Verification items for the finished model (mm, model axes). Face numbers are marked on the shaded views. A direction names the side the tool comes from. Coordinates: 2 decimals unless noted, no trailing zeros. Loops run counter-clockwise (first coordinate to the right, second up) from the corner with the lowest first, then second, coordinate; pieces in that order, holes last.
Q1. Access from +Z, -Z, +X, -X, +Y, -Y to the whole of each face (thin tool, end or side, straight path). Record for the marked faces 1, 2 and 3.
Q2. Sectioned sample at B-B (z = -46). Enter the section's corners in (x, y).
Q3. Go/stop test with flat-tipped pins: P1, Ø2, axis at y = -2.5, z = -36.5, coming from the -X side; P2, Ø16, axis at x = -39.5, z = -17.5, coming from the +Y side; P3, Ø13, axis at x = -18, y = 24.5, coming from the -Z side; P4, Ø1, axis at x = -24, y = 4.5, coming from the -Z side. Record where each tip stops, or that it passes through.
Q4. Sectioned sample at D-D (y = 12). Enter the section's corners in (x, z).
Q5. Sectioned sample at A-A (x = -46). Enter the section's corners in (y, z).
Q6. Material ranges on probe 1 along X at (y, z) = (-3.65, -46); probe 2 along Y at (x, z) = (-13, -16.5); probe 3 along Z at (x, y) = (-42, -2), recorded low to high.
Q7. Sectioned sample at C-C (x = -16.5). Enter the section's corners in (y, z).
```python
from build123d import *

# Parameters (mm, degrees)
SKETCH1_W                    = 33.7
SKETCH1_H                    = 20.3
SKETCH1_W_2                  = 20.3
SKETCH1_H_2                  = 33.7
BOSS_EXTRUDE1_DEPTH          = 24
SHELL1_T                     = -4
SKETCH2_R                    = 1
CUT_EXTRUDE1_DEPTH           = 24
SKETCH3_R                    = 4.2
CUT_EXTRUDE2_DEPTH           = 3
CUT_EXTRUDE2_DRAFT           = -45
CUT_EXTRUDE2_PROFILE_2_DEPTH = 3
CUT_EXTRUDE2_PROFILE_2_DRAFT = -45
SKETCH4_W                    = 20.3
SKETCH4_H                    = 22
BOSS_EXTRUDE2_DEPTH          = 50
SHELL2_T                     = -4
CUT_EXTRUDE3_REACH           = 93.28
SKETCH5_R                    = 1
SKETCH6_R                    = 4.2
CUT_EXTRUDE4_DEPTH           = 3
CUT_EXTRUDE4_DRAFT           = -45
CUT_EXTRUDE5_REACH           = 93.28
SKETCH7_R                    = 1
SKETCH8_R                    = 4.2
CUT_EXTRUDE6_DEPTH           = 3
CUT_EXTRUDE6_DRAFT           = -45
FILLET1_R                    = 10


with BuildPart() as part:
    # Sketch1 → Boss-Extrude1 (new body)
    with BuildSketch(Plane(origin=(0, 0, 0), x_dir=(1, 0, 0), z_dir=(0, 1, 0))):
        with Locations((-37.15, 10.15)):
            Rectangle(SKETCH1_W, SKETCH1_H)
        with Locations((-10.15, 10.15)):
            Rectangle(SKETCH1_W_2, SKETCH1_H)
        with Locations((-10.15, 37.15)):
            Rectangle(SKETCH1_W_2, SKETCH1_H_2)
    extrude(amount=-BOSS_EXTRUDE1_DEPTH)

    # Shell1
    shell1_openings = [part.faces().sort_by_distance(p)[0] for p in [
        (-53.236324676, -24, -10.15),
        (-54, -12, -10.15),
        (-37.15, -12, -20.3),
        (-20.3, -12, -37.15),
        (-10.15, -12, -54),
    ]]
    offset(amount=SHELL1_T, openings=shell1_openings, kind=Kind.INTERSECTION)

    # Sketch2 → Cut-Extrude1 (cut)
    with BuildSketch(Plane(origin=(0, 0, 0), x_dir=(1, 0, 0), z_dir=(0, 1, 0))):
        with Locations(Location((-10.15, 46, 0), (0, 0, 270))):
            Circle(SKETCH2_R)
        with Locations(Location((-46, 10.15, 0), (0, 0, 270))):
            Circle(SKETCH2_R)
    extrude(amount=-CUT_EXTRUDE1_DEPTH, mode=Mode.SUBTRACT)


with BuildPart() as cut_extrude2_tool:
    # Sketch3 → Cut-Extrude2 (with draft: the straight prism first)
    with BuildSketch(Plane(origin=(0, 0, 0), x_dir=(1, 0, 0), z_dir=(0, 1, 0))):
        with Locations((-46, 10.15)):
            Circle(SKETCH3_R)
    extrude(amount=-CUT_EXTRUDE2_DEPTH)
    # Cut-Extrude2: the draft: its side faces are tilted about the plane it starts from
    cut_extrude2_sides = [cut_extrude2_tool.faces().sort_by_distance(p)[0] for p in [
        (-50.2, -1.5, -10.15),
    ]]
    draft(cut_extrude2_sides, Plane(origin=(0, 0, 0), x_dir=(1, 0, 0), z_dir=(0, 1, 0)), CUT_EXTRUDE2_DRAFT)


with BuildPart() as part_1:
    add(part.part)

    # Cut-Extrude2: cut by cut_extrude2_tool
    add(cut_extrude2_tool.part, mode=Mode.SUBTRACT)


with BuildPart() as cut_extrude2_profile_2_tool:
    # Sketch3 → Cut-Extrude2 profile 2 (with draft: the straight prism first)
    with BuildSketch(Plane(origin=(0, 0, 0), x_dir=(1, 0, 0), z_dir=(0, 1, 0))):
        with Locations((-10.15, 46)):
            Circle(SKETCH3_R)
    extrude(amount=-CUT_EXTRUDE2_PROFILE_2_DEPTH)
    # Cut-Extrude2 profile 2: the draft: its side faces are tilted about the plane it starts from
    cut_extrude2_profile_2_sides = [cut_extrude2_profile_2_tool.faces().sort_by_distance(p)[0] for p in [
        (-14.35, -1.5, -46),
    ]]
    draft(cut_extrude2_profile_2_sides, Plane(origin=(0, 0, 0), x_dir=(1, 0, 0), z_dir=(0, 1, 0)), CUT_EXTRUDE2_PROFILE_2_DRAFT)


with BuildPart() as part_2:
    add(part_1.part)

    # Cut-Extrude2 profile 2: cut by cut_extrude2_profile_2_tool
    add(cut_extrude2_profile_2_tool.part, mode=Mode.SUBTRACT)


with BuildPart() as body_2:
    # Sketch4 → Boss-Extrude2 (new body)
    with BuildSketch(Plane(origin=(0, 0, 0), x_dir=(1, 0, 0), z_dir=(0, 1, 0))):
        with Locations((-10.15, 11)):
            Rectangle(SKETCH4_W, SKETCH4_H)
    extrude(amount=BOSS_EXTRUDE2_DEPTH)

    # Shell2
    shell2_openings = [body_2.faces().sort_by_distance(p)[0] for p in [
        (-10.15, 50, -11),
        (-10.15, 0, -11),
        (-20.3, 25, -11),
        (-10.15, 25, -22),
    ]]
    offset(amount=SHELL2_T, openings=shell2_openings, kind=Kind.INTERSECTION)


with BuildPart() as part_3:
    add(part_2.part)

    # Combine1: union body 2
    add(body_2.part)

    # Sketch5 → Cut-Extrude3 (cut, up to next)
    with BuildSketch(Plane.XY, mode=Mode.PRIVATE) as cut_extrude3_sk1:
        with Locations((-10.15, 42)):
            Circle(SKETCH5_R)
    cut_extrude3_tool1 = extrude(cut_extrude3_sk1.sketch, amount=-CUT_EXTRUDE3_REACH, mode=Mode.PRIVATE) & part_3.part
    add(cut_extrude3_tool1.solids().sort_by_distance((-10.15, 42, 0))[0], mode=Mode.SUBTRACT)


with BuildPart() as cut_extrude4_tool:
    # Sketch6 → Cut-Extrude4 (with draft: the straight prism first)
    with BuildSketch(Plane.XY):
        with Locations((-10.15, 42)):
            Circle(SKETCH6_R)
    extrude(amount=-CUT_EXTRUDE4_DEPTH)
    # Cut-Extrude4: the draft: its side faces are tilted about the plane it starts from
    cut_extrude4_sides = [cut_extrude4_tool.faces().sort_by_distance(p)[0] for p in [
        (-14.35, 42, -1.5),
    ]]
    draft(cut_extrude4_sides, Plane.XY, CUT_EXTRUDE4_DRAFT)


with BuildPart() as part_4:
    add(part_3.part)

    # Cut-Extrude4: cut by cut_extrude4_tool
    add(cut_extrude4_tool.part, mode=Mode.SUBTRACT)

    # Sketch7 → Cut-Extrude5 (cut, up to next)
    with BuildSketch(Plane(origin=(0, 0, 0), x_dir=(0, 0, -1), z_dir=(1, 0, 0)), mode=Mode.PRIVATE) as cut_extrude5_sk1:
        with Locations((11, 20)):
            Circle(SKETCH7_R)
    cut_extrude5_tool1 = extrude(cut_extrude5_sk1.sketch, amount=-CUT_EXTRUDE5_REACH, mode=Mode.PRIVATE) & part_4.part
    add(cut_extrude5_tool1.solids().sort_by_distance((0, 20, -11))[0], mode=Mode.SUBTRACT)


with BuildPart() as cut_extrude6_tool:
    # Sketch8 → Cut-Extrude6 (with draft: the straight prism first)
    with BuildSketch(Plane(origin=(0, 0, 0), x_dir=(0, 0, -1), z_dir=(1, 0, 0))):
        with Locations((11, 20)):
            Circle(SKETCH8_R)
    extrude(amount=-CUT_EXTRUDE6_DEPTH)
    # Cut-Extrude6: the draft: its side faces are tilted about the plane it starts from
    cut_extrude6_sides = [cut_extrude6_tool.faces().sort_by_distance(p)[0] for p in [
        (-1.5, 20, -6.8),
    ]]
    draft(cut_extrude6_sides, Plane(origin=(0, 0, 0), x_dir=(0, 0, -1), z_dir=(1, 0, 0)), CUT_EXTRUDE6_DRAFT)


with BuildPart() as part_5:
    add(part_4.part)

    # Cut-Extrude6: cut by cut_extrude6_tool
    add(cut_extrude6_tool.part, mode=Mode.SUBTRACT)

    # Fillet1
    fillet1_edges = [part_5.edges().sort_by_distance(p)[0] for p in [
        (-2, 0, -22),
        (-20.3, 0, -2),
    ]]
    fillet(fillet1_edges, radius=FILLET1_R)


solid = part_5.part
```
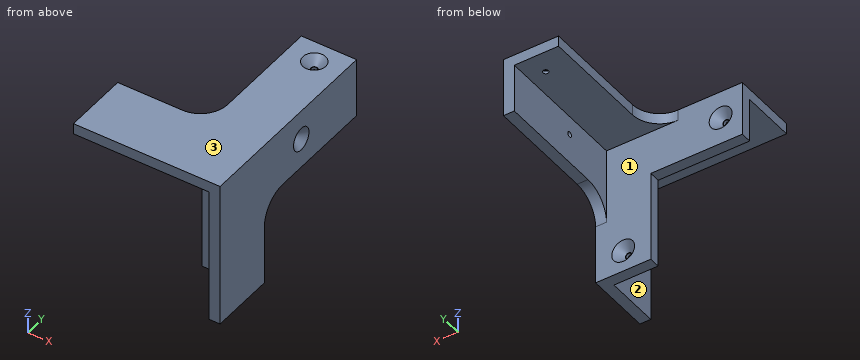
Geometry check:
1. face 1: -Z, -X, +Y
1. face 2: -Z, -X, -Y
1. face 3: +Z, +X, -X, +Y, -Y
2. outline: (-20.3, -4) - (-11.15, -4) - (-11.15, -3) - (-11.35, -3) - (-14.35, 0) - (-20.3, 0) - close; (-9.15, -4) - (-4, -4) - (-4, -24) - (0, -24) - (0, 0) - (-5.95, 0) - (-8.95, -3) - (-9.15, -3) - close
3. P1: stops at x = -20.3
3. P2: stops at y = 0
3. P3: stops at z = -4
3. P4: passes through
4. outline: (-20.3, -4) - (-4, -4) - (-4, -22) - (0, -22) - (0, 0) - (-20.3, 0) - close
5. outline: (-24, -4) - (-4, -4) - (-4, -9.15) - (-3, -9.15) - (-3, -8.95) - (0, -5.95) - (0, 0) - (-24, 0) - close; (-4, -20.3) - (0, -20.3) - (0, -14.35) - (-3, -11.35) - (-3, -11.15) - (-4, -11.15) - close
6. probe 1: x = -20.3 to -11.15, -9.15 to 0
6. probe 2: y = -4 to 0
6. probe 3: z = -20.3 to 0
7. outline: (-24, -4) - (-4, -4) - (-4, -54) - (0, -54) - (0, -4) - (50, -4) - (50, 0) - (-24, 0) - close
